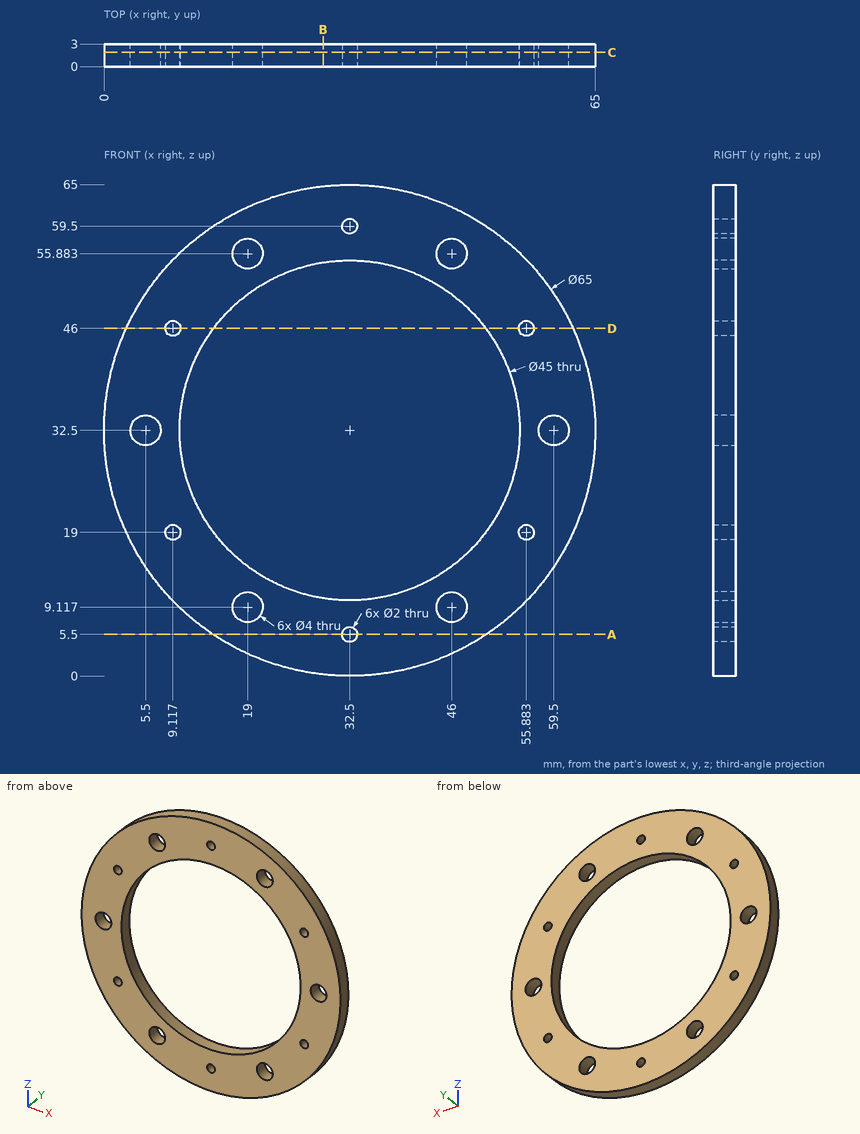
Answer from the drawing. Dimensions are ordinates in mm from the lowest x, y and z of the part. Give positions to 0.01 mm unless a question says otherwise; leave off trailing zeros. Write each loop counter-clockwise with the first axis right and the second up, starting at its lowest first coordinate (ties: lowest second). Pieces come first, ordered by that corner, then holes. Notation, with made-up numbers: M 79,25.25 L 134,25.25 A28 cw 134,54.25 Z; hole C -21,68 d4. An arc over 180 degrees is marked long. Answer as CSV lines item,"result".
Q1. Given P1, Ø4.5, axis at x = 5.5, z = 32.5, coming from the +Y side; P2, Ø1, axis at x = 57, y = 2.5, coming from the +Z side (1 decimal), each flat-ended and moving along its own axis, determine where each tip first touches the part or whether it passes through.
A:
P1,"stops at y = 3"
P2,"stops at z = 54.4"
Q2. A cutting plane is placed at D-D on z = 46. Write down the section's boundary in (x, y).
A:
outline,"M 2.94,0 L 8.12,0 L 8.12,3 L 2.94,3 Z; M 10.12,0 L 14.5,0 L 14.5,3 L 10.12,3 Z; M 50.5,0 L 54.88,0 L 54.88,3 L 50.5,3 Z; M 56.88,0 L 62.06,0 L 62.06,3 L 56.88,3 Z"
Q3. Find the intervals of material crossed by probe 1 along X at (y, z) = (1.4, 32.5); probe 2 along X at (y, z) = (2.4, 46) (1 decimal); probe 3 along X at (y, z) = (1.95, 8.5) (1 decimal), in increasing order. Write a range as [from, to].
A:
probe 1,"x = [0, 3.5], [7.5, 10], [55, 57.5], [61.5, 65]"
probe 2,"x = [2.9, 8.1], [10.1, 14.5], [50.5, 54.9], [56.9, 62.1]"
probe 3,"x = [10.6, 17.1], [20.9, 44.1], [47.9, 54.4]"
Q4. A cutting plane is placed at B-B on x = 29. Write down the section's boundary in (y, z), plus the area to 3 significant figures.
A:
outline,"M 0,0.19 L 3,0.19 L 3,10.27 L 0,10.27 Z; M 0,54.73 L 3,54.73 L 3,64.81 L 0,64.81 Z"
area,"60.5 mm²"
Q5. A cutting plane is placed at C-C on y = 1.9. Count the separate pieces of the cut face and the enclosed holes in it, plus the area to 3 significant figures.
A:
separate pieces,"1"
enclosed holes,"13"
area,"1,630 mm²"
Q6. A cutting plane is placed at A-A on z = 5.5. Write down the section's boundary in (x, y).
A:
outline,"M 14.41,0 L 31.5,0 L 31.5,3 L 14.41,3 Z; M 33.5,0 L 50.59,0 L 50.59,3 L 33.5,3 Z"
